For this review, take the finished solid that the model builds, in its own axes (mm). A direction names the side the tool comes from. Coordinates: 2 decimals unless noted, no trailing zeros. Loops run counter-clockwise (first coordinate to the right, second up) from the corner with the lowest first, then second, coordinate; pieces in that order, holes last. Notation, with made-up numbers: M 17,-22.75 L 69,-22.75 A22 cw 69,-5.75 Z; hole C -24.5,16.25 d1. An arc over 180 degrees is marked long. Answer as a JSON object with one key per item and string values. Group by question number.
Item 1: Add section C-C (y = 0). State the section outline as (x, z) points.
Item 2: Add section A-A (x = -59.5). State the section outline as (y, z) points, then the cut area to 3 significant figures.
Item 3: Add section D-D (x = -56). State the section outline as (y, z) points, then the cut area to 3 significant figures.
Item 4: Add section B-B (z = 6.5). State the section outline as (x, y) points, then the cut area to 3 significant figures.
Item 5: Wall thickness on L1, parallel to Y at x = -58.75, z = 4.5; L2, parallel to Y at x = -58.25, z = 6; L3, parallel to X at y = -4, z = 0.85: over which ranges is each line inside the solid? List them lowest first. Write a range as from..to.
Item 6: Mouldability with a two-part tool opening along Y and no side actions: class faces 3 (the face through (-54.092, -3.399, 0.986)), 4 (the face through (-55, 9, 10)), 5 (the face through (-62.527, 5.231, 4.93)) as +Y half, -Y half, draft (parallel to the pull), parting line (faces both ways), or undercut.
Item 7: Tool access review of faces 1 (the face through (-58, 6, 0)), 2 (the face through (-53.9, 3.44, 5.94)): name each direction out of +Z, -Z, +X, -X, +Y, -Y from which nothing blocks a thin tool from reaching the whole face with its end or side.
Item 8: Insertion check: pin 1 (2.5 mm diameter, centred on x = -59.13, y = 15.75, fed in from +Z); pin 2 (6 mm diameter, centred on y = 4.5, z = 4, fed in from +X); pin 3 (1.5 mm diameter, centred on y = 0, z = 7.5, fed in from -X); pin 4 (4 mm diameter, centred on y = -0.5, z = 1.5, fed in from +X). Each pin has a flat end and moves straight along its axis. Give the tip position at first contact, or say it passes through.
from build123d import *

# Parameters (mm, degrees)
SKETCH1_R           = 2
BOSS_EXTRUDE1_DEPTH = 10
CUT_EXTRUDE1_START  = -8
CUT_EXTRUDE1_DEPTH  = 8


with BuildPart() as part:
    # Sketch1 → Boss-Extrude1 (new body)
    with BuildSketch(Plane.XY):
        with BuildLine():
            Line((-64.072556879, 14.969286371), (-60.938217786, -4.783584773))
            ThreePointArc((-60.938217786, -4.783584773), (-55.216415227, -8.938217786), (-51.061782214, -3.216415227))
            Line((-51.061782214, -3.216415227), (-54.196121307, 16.536455918))
            ThreePointArc((-54.196121307, 16.536455918), (-59.917923866, 20.691088931), (-64.072556879, 14.969286371))
        make_face()
        with Locations((-59.134339093, 15.752871145)):
            Circle(SKETCH1_R, mode=Mode.SUBTRACT)
        with Locations((-56, -4)):
            Circle(SKETCH1_R, mode=Mode.SUBTRACT)
    extrude(amount=BOSS_EXTRUDE1_DEPTH)

    # Sketch2 → Cut-Extrude1 (cut)
    with BuildSketch(Plane.XY.offset(10).offset(CUT_EXTRUDE1_START)):
        with BuildLine():
            ThreePointArc((-55.686566091, -5.975287114), (-57.975287114, -4.313433909), (-56.313433909, -2.024712886))
            Line((-56.313433909, -2.024712886), (-57.567169546, 5.876435572))
            Line((-57.567169546, 5.876435572), (-58.507471274, 11.802296916))
            ThreePointArc((-58.507471274, 11.802296916), (-60.053776286, 10.912358208), (-60.613031521, 9.218167051))
            Line((-60.613031521, 9.218167051), (-59.995764214, -4.184033555))
            ThreePointArc((-59.995764214, -4.184033555), (-58.526672296, -7.100955838), (-55.373132181, -7.950574229))
            Line((-55.373132181, -7.950574229), (-55.686566091, -5.975287114))
        make_face()
        with BuildLine():
            Line((-57.567169546, 5.876435572), (-56.313433909, -2.024712886))
            ThreePointArc((-56.313433909, -2.024712886), (-54.701321406, -2.479002331), (-54, -4))
            ThreePointArc((-54, -4), (-54.479002331, -5.298678594), (-55.686566091, -5.975287114))
            Line((-55.686566091, -5.975287114), (-55.373132181, -7.950574229))
            ThreePointArc((-55.373132181, -7.950574229), (-52.637503946, -6.166476468), (-52.143539746, -2.938061061))
            Line((-52.143539746, -2.938061061), (-55.705391229, 9.996899859))
            ThreePointArc((-55.705391229, 9.996899859), (-56.761631095, 11.434748057), (-58.507471274, 11.802296916))
            Line((-58.507471274, 11.802296916), (-57.567169546, 5.876435572))
        make_face()
    extrude(amount=CUT_EXTRUDE1_DEPTH, mode=Mode.SUBTRACT)


solid = part.part
From the geometry:
{
 "1": {"outline": "M -61.7,0 L -51.57,0 L -51.57,10 L -52.95,10 L -52.95,2 L -60.19,2 L -60.19,10 L -61.7,10 Z"},
 "2": {"outline": "M -7.57,0 L 13.79,0 L 13.79,10 L 11.41,10 L 11.41,2 L -5.94,2 L -5.94,10 L -7.57,10 Z; M 17.72,0 L 20.74,0 L 20.74,10 L 17.72,10 Z", "area": "105 mm²"},
 "3": {"outline": "M -9,0 L -6,0 L -6,2 L -8,2 L -8,10 L -9,10 Z; M -2,0 L 19.65,0 L 19.65,10 L 10.67,10 L 10.67,2 L -2,2 Z", "area": "129 mm²"},
 "4": {"outline": "M -64.07,14.97 L -60.94,-4.78 A5 ccw -51.06,-3.22 L -54.2,16.54 A5 ccw Z; hole C -59.13,15.75 d4; hole M -60.61,9.22 L -60,-4.18 A4 ccw long -52.14,-2.94 L -55.71,10 A2.5 ccw Z", "area": "143 mm²"},
 "5": {"L1": "y = -8.18..-6.9, 11.75..13.79, 17.72..20.74", "L2": "y = -8.47..-7.31, 11.83..13.96, 17.55..20.67", "L3": "x = -61.06..-58, -54..-51"},
 "6": {"face 3": "undercut", "face 4": "draft", "face 5": "-Y half"},
 "7": {"face 1": "-Z, +X, -X, +Y, -Y", "face 2": "+Z"},
 "8": {"pin 1": "passes through", "pin 2": "stops at x = -51.81", "pin 3": "stops at x = -61.82", "pin 4": "stops at x = -51.18"}
}
